Check sheet for the drawn part. Datum: minimum x, y, z corner. Units: mm. A direction names the side the tool comes from. Coordinates: 2 decimals unless noted, no trailing zeros. Order: outer loops, then holes, each group sorted by start corner. A loop starts at its lowest first (then second) coordinate and runs counter-clockwise, first axis right, second up. Notation, with made-up numbers: (19, 88) - (56, 88) arc R30 cw to (56, 127) - close; hole circle Ø9 at (4, 89.25). An arc over 180 degrees is marked (long way). Return JSON: item names as keys, results as strings. Group by question number.
Item 1: Section check A-A on z = 5. Enter the section's corners in (x, y) (3 decimals), then the cut area to 3 significant figures.
Item 2: Section check D-D on x = 8.25. Enter the section's corners in (y, z), then the cut area to 3 significant figures.
Item 3: Tool access check on the marked faces 4 and 5. Record the directions out of +Z, -Z, +X, -X, +Y, -Y that give a thin tool (end or side, any length) a straight path to the whole face; none if there is none.
Item 4: Section check C-C on z = 9. Enter the section's corners in (x, y) (3 decimals), then the cut area to 3 significant figures.
Item 5: Draft check along Z on the marked faces 1, 2 and 3. Enter one of: pulls with the +Z half, pulls with the -Z half, needs draft (parallel to the pull), parting line crosses it, or undercut.
Item 6: Section check B-B on x = 3. Enter the section's corners in (y, z) (3 decimals).
Item 7: Scan lines: probe 1 along Z at (x, y) = (3, 1.2) (3 decimals); probe 2 along X at (y, z) = (1.2, 5) (3 decimals); probe 3 along X at (y, z) = (1.55, 5) (3 decimals). Record each from-to range of solid material in increasing order.
Item 8: Gauge pin test, flat ends, axial feed: pin 1 (1.8 mm diameter, centred on y = 3.5, z = 7, fed in from -X); pin 2 (4 mm diameter, centred on x = 2.5, z = 7, fed in from +Y). Record the tip position at first contact, or that the pin passes through.
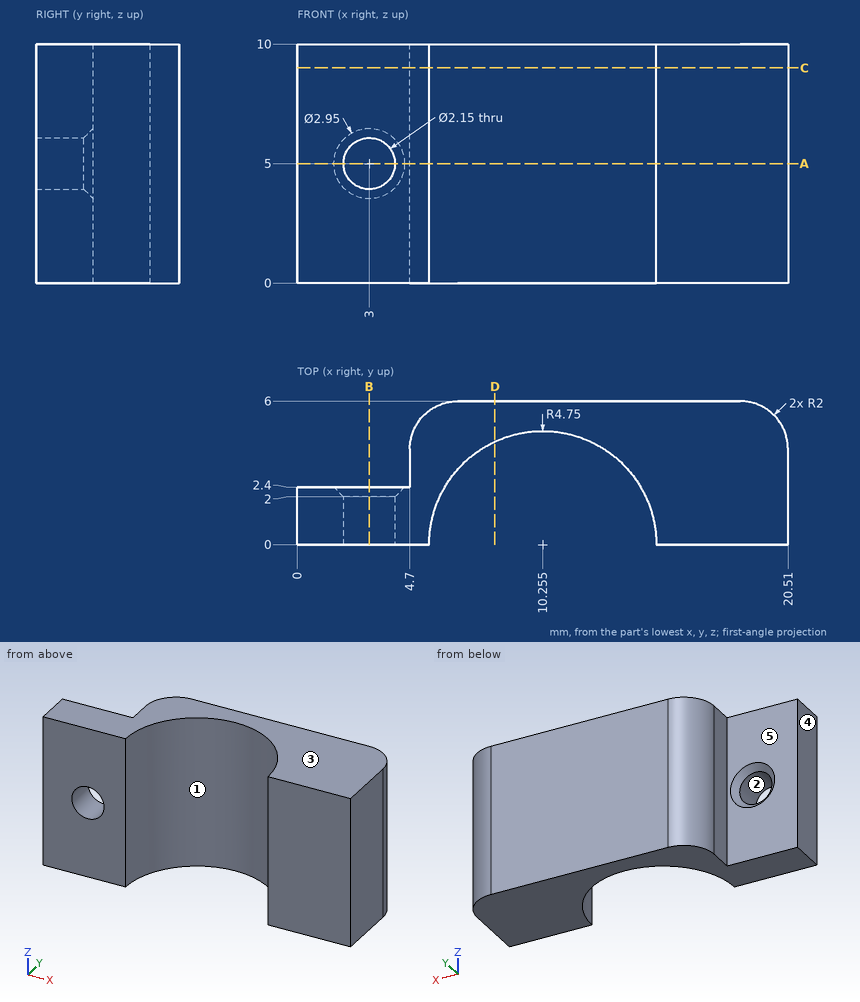
Computed:
{
 "1": {"outline": "(0, 0) - (1.925, 0) - (1.925, 2) - (1.525, 2.4) - (0, 2.4) - close; (4.075, 0) - (5.505, 0) arc R4.75 cw to (15.005, 0) - (20.51, 0) - (20.51, 4) arc R2 ccw to (18.51, 6) - (6.7, 6) arc R2 ccw to (4.7, 4) - (4.7, 2.4) - (4.475, 2.4) - (4.075, 2) - close", "area": "63.7 mm²"},
 "2": {"outline": "(4.31, 0) - (6, 0) - (6, 10) - (4.31, 10) - close", "area": "16.9 mm²"},
 "3": {"face 4": "+Z, -Z, -X, +Y, -Y", "face 5": "+Z, -Z, -X, +Y"},
 "4": {"outline": "(0, 0) - (5.505, 0) arc R4.75 cw to (15.005, 0) - (20.51, 0) - (20.51, 4) arc R2 ccw to (18.51, 6) - (6.7, 6) arc R2 ccw to (4.7, 4) - (4.7, 2.4) - (0, 2.4) - close", "area": "69.0 mm²"},
 "5": {"face 1": "needs draft", "face 2": "undercut", "face 3": "pulls with the +Z half"},
 "6": {"outline": "(0, 0) - (2.4, 0) - (2.4, 3.525) - (2, 3.925) - (0, 3.925) - close; (0, 6.075) - (2, 6.075) - (2.4, 6.475) - (2.4, 10) - (0, 10) - close"},
 "7": {"probe 1": "z = 0 to 3.925, 6.075 to 10", "probe 2": "x = 0 to 1.925, 4.075 to 5.659, 14.851 to 20.51", "probe 3": "x = 0 to 1.925, 4.075 to 5.765, 14.745 to 20.51"},
 "8": {"pin 1": "stops at x = 4.7", "pin 2": "stops at y = 2.4"}
}
